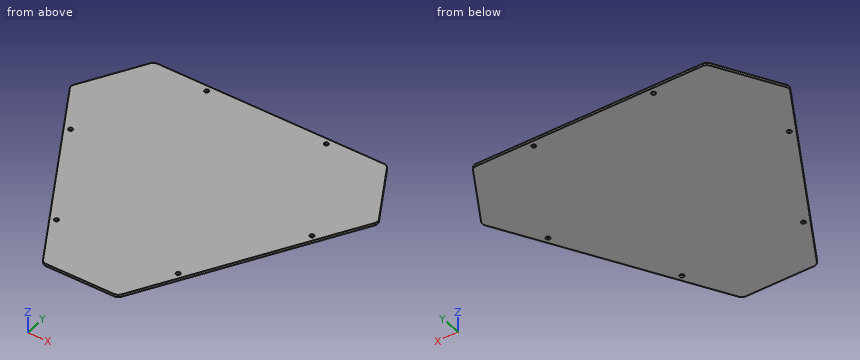
```python
from build123d import *

# Parameters (mm, degrees)
ESTRUSIONE_ESTRUSIONE1_DEPTH = 4
RACCORDO1_R                  = 10
SCHIZZO2_R                   = 3.5
TAGLIO_ESTRUSIONE1_DEPTH     = 10


with BuildPart() as part:
    # Schizzo1 → Estrusione-Estrusione1 (new body)
    with BuildSketch(Plane(origin=(0, 0, 0), x_dir=(-1, 0, 0), z_dir=(0, 0, 1))):
        Polygon((559.259871964, -2.574697247), (461.759871964, 166.300256491), (364.223704599, 335.112566514), (239.016445177, 335.112566514), (44.088779908, -2.637340962), (106.656242253, -111.007364644), (496.656242253, -111.007364644), align=None)
    extrude(amount=ESTRUSIONE_ESTRUSIONE1_DEPTH)

    # Raccordo1
    raccordo1_edges = [part.edges().sort_by_distance(p)[0] for p in [
        (-559.259871964, 2.574697247, 2),
        (-496.656242253, 111.007364644, 2),
        (-106.656242253, 111.007364644, 2),
        (-44.088779908, 2.637340962, 2),
        (-239.016445177, -335.112566514, 2),
        (-364.223704599, -335.112566514, 2),
    ]]
    fillet(raccordo1_edges, radius=RACCORDO1_R)

    # Schizzo2 → Taglio-Estrusione1 (cut)
    with BuildSketch(Plane.XY.offset(4)):
        with Locations((-503.182756728, -74.746951028)):
            Circle(SCHIZZO2_R)
        with Locations((-403.12710947, -247.919891905)):
            Circle(SCHIZZO2_R)
        with Locations((-201.661073821, 101.160104014)):
            Circle(SCHIZZO2_R)
        with Locations((-401.661063497, 101.095842135)):
            Circle(SCHIZZO2_R)
        with Locations((-200.081936903, -247.918860697)):
            Circle(SCHIZZO2_R)
        with Locations((-100.137594485, -74.681657941)):
            Circle(SCHIZZO2_R)
    extrude(amount=-TAGLIO_ESTRUSIONE1_DEPTH, mode=Mode.SUBTRACT)


solid = part.part
```
Check sheet for the modelled part. Datum: model origin and axes. Units: mm. Round coordinates to 2 decimals unless told otherwise and drop trailing zeros. Loops run counter-clockwise (first coordinate to the right, second up) from the corner with the lowest first, then second, coordinate; pieces in that order, holes last. Notation, with made-up numbers: (-35, -12.75) -> (10, -12.75) arc R18 cw to (10, 20.25) -> close; hole circle Ø9 at (-6.75, -7). An arc over 180 degrees is marked (long way). Answer in a Markdown table with one row per item.
Q1. Sectioned sample at C-C on y = -297.5. Enter the section's corners in (x, z), then the cut area to 3 significant figures.
Data:
| item | result |
|---|---|
| outline | (-385.96, 0) -> (-217.31, 0) -> (-217.31, 4) -> (-385.96, 4) -> close |
| area | 675 mm^2 |
Q2. Sectioned sample at B-B on x = -160.5. Enter the section's corners in (y, z), then the cut area to 3 significant figures.
Data:
| item | result |
|---|---|
| outline | (-199.07, 0) -> (111.01, 0) -> (111.01, 4) -> (-199.07, 4) -> close |
| area | 1,240 mm^2 |
Q3. Thickness scan on L1, parallel to X at y = -74.5, z = 0.4; L2, parallel to X at y = -247, z = 2.3; L3, parallel to X at y = 1, z = 3.2. Record the ranges inside material, lowest first.
Data:
| item | result |
|---|---|
| L1 | x = -514.76 to -506.67, -499.69 to -103.63, -96.64 to -88.61 |
| L2 | x = -415.13 to -406.5, -399.75 to -203.46, -196.7 to -188.16 |
| L3 | x = -557.59 to -45.77 |
Q4. Sectioned sample at A-A on z = 1.75. Enter the section's corners in (x, y) (1 decimal).
Data:
| item | result |
|---|---|
| outline | (-556.4, -2.4) -> (-461.8, -166.3) -> (-367.1, -330.1) arc R10 ccw to (-358.5, -335.1) -> (-244.8, -335.1) arc R10 ccw to (-236.1, -330.1) -> (-47, -2.4) arc R10 ccw to (-47, 7.6) -> (-103.8, 106) arc R10 ccw to (-112.4, 111) -> (-490.9, 111) arc R10 ccw to (-499.5, 106) -> (-556.4, 7.6) arc R10 ccw to start; hole circle Ø7 at (-503.2, -74.7); hole circle Ø7 at (-403.1, -247.9); hole circle Ø7 at (-401.7, 101.1); hole circle Ø7 at (-201.7, 101.2); hole circle Ø7 at (-200.1, -247.9); hole circle Ø7 at (-100.1, -74.7) |
Q5. Go/stop test with flat-tipped pins: P1, Ø2, axis at x = -200.5, z = 2, coming from the -Y side; P2, Ø6.5, axis at x = -503.18, y = -74.75, coming from the +Z side (3 decimals); P3, Ø2, axis at y = -149.5, z = 2.5, coming from the -X side; P4, Ø2, axis at y = 23.5, z = 2, coming from the -X side. Record where each tip stops, or that it passes through.
Data:
| item | result |
|---|---|
| P1 | stops at y = -270.11 |
| P2 | passes through |
| P3 | stops at x = -472.04 |
| P4 | stops at x = -547.76 |
